Autodesk Inventor part; units mm, degrees
ref_plane "YZ Plane" through (0, 0, 0) normal (1, 0, 0) x (0, 1, 0)
ref_plane "XZ Plane" through (0, 0, 0) normal (0, 1, 0) x (-1, 0, 0)
ref_plane "XY Plane" through (0, 0, 0) normal (0, 0, 1) x (1, 0, 0)
sketch "Sketch1" plane through (0, 0, 0) normal (0, 1, 0) x (-1, 0, 0)
  line L0 (-5.422, -5) -> (5.422, -5)
  line L1 (10.422, 0) -> (10.422, 0)
  line L2 (5.422, 5) -> (-5.422, 5)
  line L3 (-10.422, 0) -> (-10.422, 0)
  line L4 (-10.422, -5) -> (10.422, 5) construction
  line L5 (10.422, -5) -> (-10.422, 5) construction
  circle A0 centre (5.422, 0) radius 2.5
  circle A1 centre (-5.422, 0) radius 2.5
  arc A2 (5.422, -5) -> (10.422, 0) centre (5.422, 0) ccw
  arc A3 (10.422, 0) -> (5.422, 5) centre (5.422, 0) ccw
  arc A4 (-5.422, 5) -> (-10.422, 0) centre (-5.422, 0) ccw
  arc A5 (-10.422, 0) -> (-5.422, -5) centre (-5.422, 0) ccw
  point P0 (0, 0)
  point P1 (10.422, 0)
  point P2 (-10.422, 0)
  dimension "d0" = 10
  dimension "d1" = 20.844
  dimension "d3" = 5
  dimension "d4" = 5
  dimension "d5" = 5
  dimension "d6" = 5
  dimension "d7" = 5
  dimension "d8" = 5
  dimension "d9" = 5
extrude "Extrusion1" add sketch "Sketch1" along normal blind 5
properties part number "link"
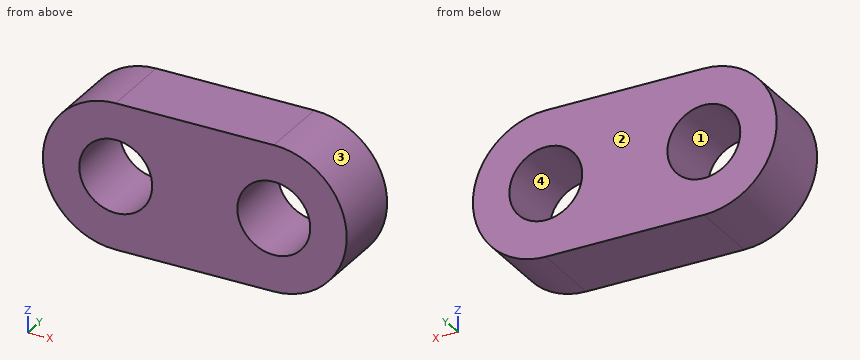
Part model, mm, in its own coordinate system. Face numbers are marked on the shaded views. Give positions to 0.01 mm unless a question says otherwise; leave off trailing zeros. Write each loop counter-clockwise with the first axis right and the second up, starting at its lowest first coordinate (ties: lowest second). Pieces come first, ordered by that corner, then holes.
1) Cut at B-B on x = -7. Write the cut outline in (y, z), then the cut area to 3 significant figures.
Resolved:
outline: (0, -4.74) - (5, -4.74) - (5, -1.94) - (0, -1.94) - close; (0, 1.94) - (5, 1.94) - (5, 4.74) - (0, 4.74) - close
area: 28.1 mm2
2) Cut at A-A on z = 0. Write the cut outline in (x, y), then the cut area to 3 significant figures.
Resolved:
outline: (-10.42, 0) - (-7.92, 0) - (-7.92, 5) - (-10.42, 5) - close; (-2.92, 0) - (2.92, 0) - (2.92, 5) - (-2.92, 5) - close; (7.92, 0) - (10.42, 0) - (10.42, 5) - (7.92, 5) - close
area: 54.2 mm2
3) Cut at D-D on z = 4.25. Write the cut outline in (x, y), then the cut area to 3 significant figures.
Resolved:
outline: (-8.06, 0) - (8.06, 0) - (8.06, 5) - (-8.06, 5) - close
area: 80.6 mm2
4) Pin check, flat tips, straight feed: pin 1 (2 mm diameter, centred on x = 8, y = 1, fed in from +Z); pin 2 (6 mm diameter, centred on x = 5.422, z = 0, fed in from -Y). Stop position of each tip, or through.
Resolved:
pin 1: stops at z = 4.74
pin 2: stops at y = 0
5) Probe L1, parallel to X at y = 3.75, z = -0.5; L2, parallel to X at y = 2.35, z = 1.75; L3, parallel to Z at x = -6.5, y = 3.6. List the from-to ranges inside material, lowest first.
Resolved:
L1: x = -10.4 to -7.87, -2.97 to 2.97, 7.87 to 10.4
L2: x = -10.11 to -7.21, -3.64 to 3.64, 7.21 to 10.11
L3: z = -4.88 to -2.26, 2.26 to 4.88
6) Cut at C-C on y = 2.25. Write the cut outline in (x, z), then the cut area to 3 significant figures.
Resolved:
outline: (-5.42, -5) - (5.42, -5) arc R5 ccw to (5.42, 5) - (-5.42, 5) arc R5 ccw to start; hole circle Ø5 at (-5.42, 0); hole circle Ø5 at (5.42, 0)
area: 148 mm2
7) Two-plate mould, pull along Z, no slides. Class the marked faces 1, 2, 3 and 4: released by +Z, released by -Z, zero draft, split by the parting line, or undercut.
Resolved:
face 1: undercut
face 2: zero draft
face 3: split by the parting line
face 4: undercut
